```python
from build123d import *

# Parameters (mm, degrees)
BLANKSKE_W         = 140
BLANKSKE_H         = 18
BLANK_DEPTH        = 15
TOOTHCUTSIM_DEPTH  = 142.947173272
TEETHCUTS_COUNT    = 19
TEETHCUTS_PITCH    = 7.853981625
SKETCH1_W          = 155.727496732
SKETCH1_H          = 72.883147076
CUT_EXTRUDE2_DEPTH = 2


with BuildPart() as part:
    # BlankSke → Blank (new body)
    with BuildSketch(Plane.XY):
        with Locations((70, 9)):
            Rectangle(BLANKSKE_W, BLANKSKE_H)
    extrude(amount=-BLANK_DEPTH)

    # TooCutSkeSim → ToothCutSim (cut, through all)
    with BuildSketch(Plane.XY):
        Polygon((1.087088424, 12.375), (-1.087088424, 12.375), (-3.143665836, 18.0254), (3.143665836, 18.0254), align=None)
    toothcutsim = extrude(amount=-TOOTHCUTSIM_DEPTH, mode=Mode.SUBTRACT)

    # TeethCuts: ToothCutSim ×19
    with Locations(*[(i * TEETHCUTS_PITCH, 0, 0) for i in range(1, TEETHCUTS_COUNT)]):
        add(toothcutsim, mode=Mode.SUBTRACT)

    # Sketch1 → Cut-Extrude2 (cut)
    with BuildSketch(Plane.XY.offset(-15)):
        with Locations((71.044371672, 7.444354081)):
            Rectangle(SKETCH1_W, SKETCH1_H)
    extrude(amount=CUT_EXTRUDE2_DEPTH, mode=Mode.SUBTRACT)


solid = part.part
```
Model file for the job. Use its own axes, mm. Give positions to 0.01 mm unless a question says otherwise; leave off trailing zeros.
1) Mould opens along X. For faces 1 (the flat face through (0, 6, -6)), 2 (the flat face through (31, 12.375, -6)), 3 (the flat face through (69, 0, -6)) say: +X half, -X half, draft (parallel to the pull), parting line (faces both ways), or undercut.
2) Saw through at A-A, the plane y = 15. Count the separate pieces of the cut face and the enclosed holes in it, then the cut area to 3 significant figures.
3) Wall check: probe 1 along Y at (x, z) = (78, -7.5) (3 decimals). Give the ranges that are in metal, low to high.
4) Pin check, flat tips, straight feed: pin 1 (0.7 mm diameter, centred on x = 133.5, z = -9, fed in from +Y) (3 decimals); pin 2 (1 mm diameter, centred on x = 56, z = -3, fed in from -Y). Stop position of each tip, or through.
Computed:
1. face 1: -X half
1. face 2: undercut
1. face 3: draft
2. separate pieces: 18
2. enclosed holes: 0
2. area: 882 mm2
3. probe 1: y = 0 to 12.375
4. pin 1: stops at y = 12.375
4. pin 2: stops at y = 0
